```python
from build123d import *

# Parameters (mm, degrees)
SKETCH1_W           = 88.9
SKETCH1_H           = 12.7
SKETCH1_R           = 3
SKETCH1_W_2         = 50.8
SKETCH1_H_2         = 5
BOSS_EXTRUDE1_DEPTH = 1.5


with BuildPart() as part:
    # Sketch1 → Boss-Extrude1 (new body, symmetric)
    with BuildSketch(Plane.XY):
        with Locations((36.83, 0)):
            Rectangle(SKETCH1_W, SKETCH1_H)
        Circle(SKETCH1_R, mode=Mode.SUBTRACT)
        with Locations((43.18, 0)):
            Rectangle(SKETCH1_W_2, SKETCH1_H_2, mode=Mode.SUBTRACT)
    extrude(amount=BOSS_EXTRUDE1_DEPTH, both=True)


solid = part.part
```
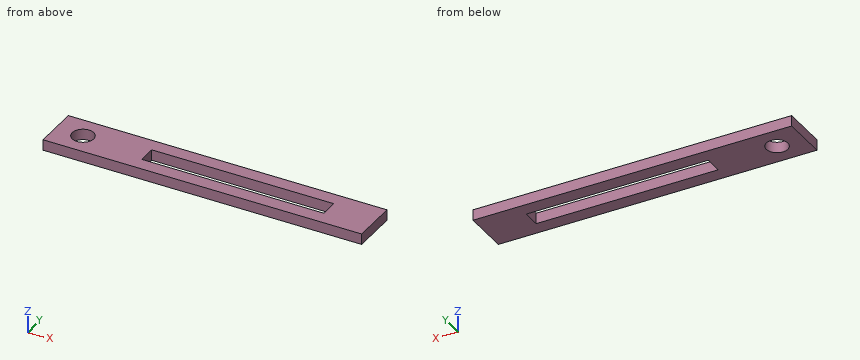
Input: part model. Units: mm. Frame: model coordinates. Coordinates: 2 decimals unless noted, no trailing zeros. Loops run counter-clockwise (first coordinate to the right, second up) from the corner with the lowest first, then second, coordinate; pieces in that order, holes last. Notation, with made-up numbers: M 56.25,1.5 L 61.25,1.5 A22 cw 61.25,12.5 Z; hole C 38.5,58 d11. An arc over 180 degrees is marked long. Answer in a Markdown table with one row per item.
1. Section C-C, the plane y = 0. Output: boundary loops of the cut face in (x, z), then the cut area to 3 significant figures.
Response:
| item | result |
|---|---|
| outline | M -7.62,-1.5 L -3,-1.5 L -3,1.5 L -7.62,1.5 Z; M 3,-1.5 L 17.78,-1.5 L 17.78,1.5 L 3,1.5 Z; M 68.58,-1.5 L 81.28,-1.5 L 81.28,1.5 L 68.58,1.5 Z |
| area | 96.3 mm2 |
2. Material intervals for line 1 (Y direction, x = 44, z = -0.15); line 2 (Y direction, x = 0, z = 0.2); line 3 (X direction, y = -1.5, z = -0.9), sorted ascending.
Response:
| item | result |
|---|---|
| line 1 | y = -6.35 to -2.5, 2.5 to 6.35 |
| line 2 | y = -6.35 to -3, 3 to 6.35 |
| line 3 | x = -7.62 to -2.6, 2.6 to 17.78, 68.58 to 81.28 |
3. Section B-B, the plane z = -0.35. Output: boundary loops of the cut face in (x, y).
Response:
| item | result |
|---|---|
| outline | M -7.62,-6.35 L 81.28,-6.35 L 81.28,6.35 L -7.62,6.35 Z; hole C 0,0 d6; hole M 17.78,-2.5 L 68.58,-2.5 L 68.58,2.5 L 17.78,2.5 Z |
4. Section A-A, the plane x = 40.5. Output: boundary loops of the cut face in (y, z), then the cut area to 3 significant figures.
Response:
| item | result |
|---|---|
| outline | M -6.35,-1.5 L -2.5,-1.5 L -2.5,1.5 L -6.35,1.5 Z; M 2.5,-1.5 L 6.35,-1.5 L 6.35,1.5 L 2.5,1.5 Z |
| area | 23.1 mm2 |
5. Section D-D, the plane x = 0. Output: boundary loops of the cut face in (y, z).
Response:
| item | result |
|---|---|
| outline | M -6.35,-1.5 L -3,-1.5 L -3,1.5 L -6.35,1.5 Z; M 3,-1.5 L 6.35,-1.5 L 6.35,1.5 L 3,1.5 Z |
